Model file for the job. Use its own axes, mm. A direction names the side the tool comes from. Coordinates: 2 decimals unless noted, no trailing zeros. Order: outer loops, then holes, each group sorted by start corner. A loop starts at its lowest first (then second) coordinate and runs counter-clockwise, first axis right, second up.
from build123d import *

# Parameters (mm, degrees)
SALIENTE_EXTRUIR1_DEPTH    = 10
CROQUIS4_R                 = 3.81
CORTAR_EXTRUIR1_DEPTH      = 61.468
CORTAR_EXTRUIR1_DEPTH_BACK = 64.008


with BuildPart() as part:
    # Croquis2 → Saliente-Extruir1 (new body)
    with BuildSketch(Plane.XY):
        with BuildLine():
            Line((-51.279919423, -17.994736431), (-56.441706153, -38.125704677))
            ThreePointArc((-56.441706153, -38.125704677), (-56.611211976, -41.10511644), (-55.639925501, -43.92685868))
            Line((-55.639925501, -43.92685868), (-33.368069091, -82.317782173))
            Line((-33.368069091, -82.317782173), (-22.449197371, -85.11749287))
            Line((-22.449197371, -85.11749287), (-28.956418222, -110.495654186))
            ThreePointArc((-28.956418222, -110.495654186), (-28.120578041, -116.354933217), (-23.386413845, -119.907040892))
            Line((-23.386413845, -119.907040892), (-15.596975427, -121.904332794))
            ThreePointArc((-15.596975427, -121.904332794), (-16.177038504, -104.258895505), (-8.511603611, -88.354838218))
            Line((-8.511603611, -88.354838218), (-39.670979585, -41.190293696))
            Line((-39.670979585, -41.190293696), (6.890267505, -10.429487701))
            ThreePointArc((6.890267505, -10.429487701), (10.624002053, 6.586393579), (-6.277032388, 10.809665323))
            Line((-6.277032388, 10.809665323), (-47.67245646, -13.22812029))
            ThreePointArc((-47.67245646, -13.22812029), (-49.955399161, -15.248752476), (-51.279919423, -17.994736431))
        make_face()
    extrude(amount=SALIENTE_EXTRUIR1_DEPTH)

    # Croquis4 → Cortar-Extruir1 (cut, two sides)
    with BuildSketch(Plane.XY) as cortar_extruir1_sk:
        Circle(CROQUIS4_R)
        with Locations((-39.080143485, -22.972272641)):
            Circle(CROQUIS4_R)
    extrude(amount=CORTAR_EXTRUIR1_DEPTH, mode=Mode.SUBTRACT)
    extrude(cortar_extruir1_sk.sketch, amount=-CORTAR_EXTRUIR1_DEPTH_BACK, mode=Mode.SUBTRACT)


solid = part.part
Q1. Cut at C-C, the plane y = 0. List the corners of the cut face in (x, z).
Established:
outline: (-24.89, 0) - (-3.81, 0) - (-3.81, 10) - (-24.89, 10) - close; (3.81, 0) - (12.5, 0) - (12.5, 10) - (3.81, 10) - close
Q2. Cut at D-D, the plane y = -101.5. List the corners of the cut face in (x, z), plus the area to 3 significant figures.
Established:
outline: (-26.65, 0) - (-15.48, 0) - (-15.48, 10) - (-26.65, 10) - close
area: 112 mm2
Q3. Drop flat-ended pins along their axis: P1, Ø3, axis at y = -9, z = 3.5, coming from the -X side; P2, Ø4.5, axis at x = -39.08, y = -22.97, coming from the -Z side; P3, Ø6, axis at x = -32.5, z = 4.5, coming from the +Y side; P4, Ø2, axis at y = -28.5, z = 5.5, coming from the -X side. Give the stop position or say it passes through.
Established:
P1: stops at x = -42.97
P2: passes through
P3: stops at y = -2.68
P4: stops at x = -54.23
Q4. Cut at B-B, the plane z = 8. List the corners of the cut face in (x, y).
Established:
outline: (-56.44, -38.13) arc R7.73 ccw to (-55.64, -43.93) - (-33.37, -82.32) - (-22.45, -85.12) - (-28.96, -110.5) arc R7.73 ccw to (-23.39, -119.91) - (-15.6, -121.9) arc R36.99 cw to (-8.51, -88.35) - (-39.67, -41.19) - (6.89, -10.43) arc R12.5 ccw to (-6.28, 10.81) - (-47.67, -13.23) arc R7.73 ccw to (-51.28, -17.99) - close; hole circle Ø7.62 at (-39.08, -22.97); hole circle Ø7.62 at (0, 0)
Q5. Probe line 1 (Y direction, x = -38, z = 9.5); line 2 (X direction, y = -1.5, z = 3.25); line 3 (X direction, y = -21.5, z = 8). List the from-to ranges inside material, lowest first.
Established:
line 1: y = -74.33 to -43.72, -40.09 to -26.63, -19.32 to -7.61
line 2: x = -27.48 to -3.5, 3.5 to 12.41
line 3: x = -52.18 to -42.59, -35.57 to -9.87
Q6. Mould opens along X. For faces 1 (the face through (-49.929, -15.215, 4.93)), 2 (the face through (-23.873, -65.103, 4.93)), 3 (the face through (-0.83, -3.72, 4.93)), 4 (the face through (-37.03, -19.76, 4.93)) say: pulls with the +X half, pulls with the -X half, needs draft (parallel to the pull), parting line crosses it, or undercut.
Established:
face 1: pulls with the -X half
face 2: pulls with the +X half
face 3: undercut
face 4: undercut
Q7. Which spindle directions (+Z, -Z, +X, -X, +Y, -Y) get a long thin tool onto all of the face, cutting with end or side? Do faces 5 (the face through (-16.72, -26.03, 4.93)), 6 (the face through (-53.825, -27.919, 4.93)), 7 (the face through (-25.657, -97.629, 4.93)). Say none if no direction does.
Established:
face 5: +Z, -Z, +X
face 6: +Z, -Z, -X, +Y
face 7: +Z, -Z, -X
Q8. Cut at A-A, the plane x = 0. List the corners of the cut face in (y, z).
Established:
outline: (-14.98, 0) - (-3.81, 0) - (-3.81, 10) - (-14.98, 10) - close; (3.81, 0) - (12.5, 0) - (12.5, 10) - (3.81, 10) - close
